Model file for the job. Use its own axes, mm. Face numbers are marked on the shaded views. A direction names the side the tool comes from. Coordinates: 2 decimals unless noted, no trailing zeros. Write each loop counter-clockwise with the first axis right and the second up, starting at its lowest first coordinate (ties: lowest second). Pieces come first, ordered by that corner, then holes. Notation, with made-up numbers: (68.5, 65.5) -> (85.5, 65.5) arc R23 ccw to (85.5, 75.5) -> close; hole circle Ø3 at (26.5, 30). An arc over 180 degrees is marked (long way). Write item = value, one per line. Start each with the question number.
Autodesk Inventor part; units mm, degrees
ref_plane "YZ Plane" through (0, 0, 0) normal (1, 0, 0) x (0, 1, 0)
ref_plane "XZ Plane" through (0, 0, 0) normal (0, 1, 0) x (-1, 0, 0)
ref_plane "XY Plane" through (0, 0, 0) normal (0, 0, 1) x (1, 0, 0)
sketch "Sketch1" plane through (0, 0, 0) normal (0, 0, 1) x (1, 0, 0)
  line L0 (0, 0) -> (3.175, 0)
  line L1 (3.175, 0) -> (3.175, 25.4)
  line L2 (3.175, 25.4) -> (0, 25.4)
  line L3 (0, 25.4) -> (0, 0)
  line L4 (0, 0) -> (25.4, 0)
  line L5 (25.4, 0) -> (25.4, 3.175)
  line L6 (25.4, 3.175) -> (0, 3.175)
  line L7 (0, 3.175) -> (0, 0)
  dimension "d0" = 3.175
  dimension "d1" = 25.4
  dimension "d2" = 25.4
  dimension "d3" = 3.175
extrude "Extrusion1" add sketch "Sketch1" along normal blind 25.4
sketch "Sketch2" plane through (3.175, 3.175, 0) normal (1, 0, 0) x (0, 0, -1)
  line L0 (0, 22.225) -> (-25.4, 22.225) construction
  line L1 (-12.7, 22.225) -> (-12.7, 9.525) construction
  circle A0 centre (-12.7, 9.525) radius 2.5797
  point P0 (0, -3.175)
  dimension "d6" = 12.7
  dimension "d7" = 5.1594
extrude "Extrusion2" cut sketch "Sketch2" against normal blind 25.4
sketch "Sketch3" plane through (3.175, 3.175, 0) normal (0, 1, 0) x (1, 0, 0)
  line L0 (-3.175, 0) -> (-3.175, -25.4) construction
  line L1 (-3.175, -12.7) -> (14.9098, -12.7) construction
  circle A0 centre (14.9098, -12.7) radius 2.5797
  dimension "d10" = 18.0848
  dimension "d11" = 5.1594
extrude "Extrusion3" cut sketch "Sketch3" against normal blind 25.4
properties part number "L-Bracket Gearbox"
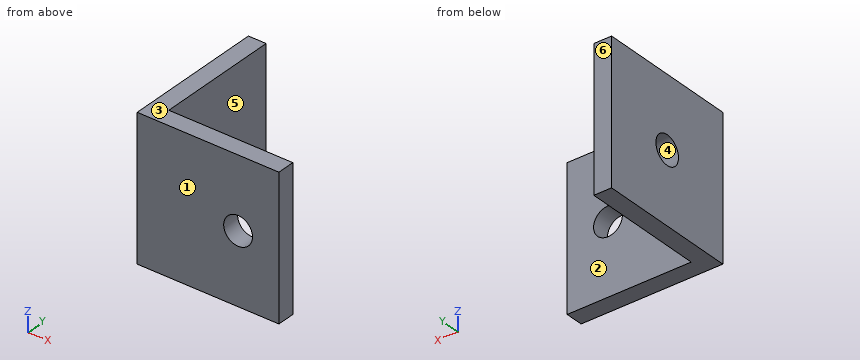
(1) Drop flat-ended pins along their axis: pin 1 Ø6 at (y, z) = (10, 6) entering from +X (3 decimals); pin 2 Ø1 at (y, z) = (22.5, 16) entering from -X; pin 3 Ø6.5 at (x, z) = (18.08, 12.7) entering from +Y (3 decimals). Give the stop position or say it passes through.
(2) Saw through at B-B (z = 14.5). Give the cut face in (x, y) (3 decimals), then the cut area to 3 significant figures.
(3) Mould opens along Y. For the marked faces 1, 2, 3 and 4 say: released by +Y, released by -Y, zero draft, split by the parting line, or undercut.
(4) Saw through at D-D (y = 2.5). Give the cut face in (x, z), then the cut area to 3 significant figures.
(5) Saw through at A-A (y = 12.7). Give the cut face in (x, z) (3 decimals).
(6) Drill centre lines: line 1 along Y through (x, z) = (1.5, 12.7); line 2 along X through (y, z) = (1.1, 12.7); line 3 along Y through (x, z) = (17.75, 7.5) (3 decimals). Where is each one in solid material? Low to high.
(7) 3-axis set-ups, long thin cutter, end or side, ignore diameter. For the marked faces 5 and 6: which of +Z, -Z, +X, -X, +Y, -Y reach the whole face in a straight line?
(8) Saw through at C-C (x = 2). Give the cut face in (y, z), then the cut area to 3 significant figures.
Returned:
q1.pin_1 = 3.175
q1.pin_2 = 0
q1.pin_3 = 3.175
q2.outline = (0, 0) -> (16.237, 0) -> (16.237, 3.175) -> (3.175, 3.175) -> (3.175, 10.852) -> (0, 10.852) -> close; (0, 14.548) -> (3.175, 14.548) -> (3.175, 25.4) -> (0, 25.4) -> close; (19.933, 0) -> (25.4, 0) -> (25.4, 3.175) -> (19.933, 3.175) -> close
q2.area = 128 mm2
q3.face_1 = released by -Y
q3.face_2 = released by +Y
q3.face_3 = zero draft
q3.face_4 = undercut
q4.outline = (0, 0) -> (25.4, 0) -> (25.4, 25.4) -> (0, 25.4) -> close; hole circle Ø5.16 at (18.08, 12.7)
q4.area = 624 mm2
q5.outline = (0, 0) -> (3.175, 0) -> (3.175, 10.12) -> (0, 10.12) -> close; (0, 15.28) -> (3.175, 15.28) -> (3.175, 25.4) -> (0, 25.4) -> close
q6.line_1 = 0 to 10.12, 15.28 to 25.4
q6.line_2 = 0 to 15.51, 20.66 to 25.4
q6.line_3 = 0 to 3.175
q7.face_5 = +Z, -Z, +X, +Y
q7.face_6 = +Z, -Z, +X, -X, +Y
q8.outline = (0, 0) -> (25.4, 0) -> (25.4, 25.4) -> (0, 25.4) -> close; hole circle Ø5.16 at (12.7, 12.7)
q8.area = 624 mm2
